Geometry check sheet. Reference: the model listing, model coordinates, mm. Face numbers are marked on the shaded views. A direction names the side the tool comes from. Coordinates: 2 decimals unless noted, no trailing zeros. Order: outer loops, then holes, each group sorted by start corner. A loop starts at its lowest first (then second) coordinate and runs counter-clockwise, first axis right, second up. Notation, with made-up numbers: (-5.5, 42) -> (52.5, 42) arc R9 ccw to (52.5, 53) -> close; hole circle Ø3 at (-39.75, 3). An arc over 180 degrees is marked (long way). Answer in a Markdown table with one row per item. Add a question column.
```python
from build123d import *

# Parameters (mm, degrees)
SCHIZZO1_W                   = 20
SCHIZZO1_H                   = 18
SCHIZZO1_R                   = 2.5
ESTRUSIONE_ESTRUSIONE1_DEPTH = 5
SCHIZZO2_W                   = 30
SCHIZZO2_H                   = 3.5
ESTRUSIONE_ESTRUSIONE2_DEPTH = 18
RACCORDO2_R                  = 1
SCHIZZO3_R                   = 2.5
TAGLIO_ESTRUSIONE1_DEPTH     = 10


with BuildPart() as part:
    # Schizzo1 → Estrusione-Estrusione1 (new body)
    with BuildSketch(Plane.XY):
        Rectangle(SCHIZZO1_W, SCHIZZO1_H)
        Circle(SCHIZZO1_R, mode=Mode.SUBTRACT)
    extrude(amount=ESTRUSIONE_ESTRUSIONE1_DEPTH)

    # Schizzo2 → Estrusione-Estrusione2 (add, through all)
    with BuildSketch(Plane.XZ.offset(9)):
        with Locations((20, 6.75)):
            Rectangle(SCHIZZO2_W, SCHIZZO2_H)
        with Locations((-20, 6.75)):
            Rectangle(SCHIZZO2_W, SCHIZZO2_H)
    extrude(amount=-ESTRUSIONE_ESTRUSIONE2_DEPTH)

    # Raccordo2
    raccordo2_edges = [part.edges().sort_by_distance(p)[0] for p in [
        (-10, 0, 5),
        (-5, 0, 5),
        (-5, 0, 8.5),
        (5, 0, 5),
        (5, 0, 8.5),
        (10, 0, 5),
        (-10, 0, 0),
        (10, 0, 0),
    ]]
    fillet(raccordo2_edges, radius=RACCORDO2_R)

    # Schizzo3 → Taglio-Estrusione1 (cut)
    with BuildSketch(Plane.XY.offset(8.5)):
        with Locations((-25, 0)):
            Circle(SCHIZZO3_R)
        with Locations((25, 0)):
            Circle(SCHIZZO3_R)
        with BuildLine():
            Line((25, 9), (35, 9))
            Line((35, 9), (35, -9))
            Line((35, -9), (25, -9))
            ThreePointArc((25, -9), (34, 0), (25, 9))
        make_face()
        with BuildLine():
            Line((-35, 9), (-35, -9))
            Line((-35, -9), (-25, -9))
            ThreePointArc((-25, -9), (-34, 0), (-25, 9))
            Line((-25, 9), (-35, 9))
        make_face()
    extrude(amount=-TAGLIO_ESTRUSIONE1_DEPTH, mode=Mode.SUBTRACT)


solid = part.part
```
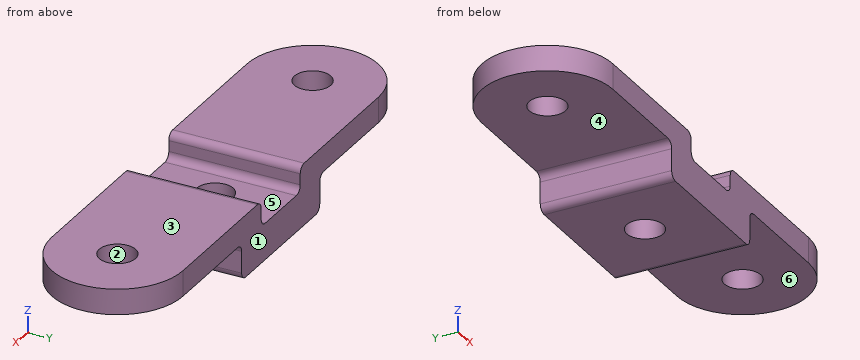
(1) Mould release check, pull along Y, two halves, no side actions. Record for the marked faces 1, 2 and 3: +Y half, -Y half, draft (parallel to the pull), parting line (faces both ways), or undercut.
(2) Cross-section at A-A (x = 0). Enter the section's corners in (y, z), plus the area to 3 significant figures.
(3) Access from +Z, -Z, +X, -X, +Y, -Y to the whole of each face (thin tool, end or side, straight path). Record for the marked faces 4, 5 and 6.
(4) Cross-section at B-B (y = 0). Give the number of separate pieces and of enclosed holes in the cut face, plus the area to 3 significant figures.
(5) Cross-section at D-D (y = -6). Enter the section's corners in (x, z).
(6) Cross-section at C-C (x = 17.5). Enter the section's corners in (y, z), plus the area to 3 significant figures.
(7) Go/stop test with flat-tipped pins: P1, Ø9, axis at x = 22, y = 2.5, coming from the -Z side; P2, Ø2.5, axis at y = -3, z = 2, coming from the +X side; P3, Ø0.8, axis at y = -3, z = 7, coming from the -X side. Record where each tip stops, or that it passes through.
(8) Scan lines: line 1 along Y through (x, z) = (0, 3.25); line 2 along X through (y, z) = (-5.75, 2.5); line 3 along Z through (x, y) = (23, -3.5). Record each from-to range of solid material in increasing order.
Checks:
| question | item | result |
|---|---|---|
| 1 | face 1 | +Y half |
| 1 | face 2 | undercut |
| 1 | face 3 | draft |
| 2 | outline | (-9, 0) -> (-2.5, 0) -> (-2.5, 5) -> (-9, 5) -> close; (2.5, 0) -> (9, 0) -> (9, 5) -> (2.5, 5) -> close |
| 2 | area | 65.0 mm² |
| 3 | face 4 | -Z, -X, +Y, -Y |
| 3 | face 5 | +Z, +Y, -Y |
| 3 | face 6 | -Z, +X, +Y, -Y |
| 4 | separate pieces | 4 |
| 4 | enclosed holes | 0 |
| 4 | area | 243 mm² |
| 5 | outline | (-31.71, 5) -> (-11, 5) arc R1 cw to (-10, 4) -> (-10, 1) arc R1 ccw to (-9, 0) -> (9, 0) arc R1 ccw to (10, 1) -> (10, 4) arc R1 cw to (11, 5) -> (31.71, 5) -> (31.71, 8.5) -> (6, 8.5) arc R1 ccw to (5, 7.5) -> (5, 6) arc R1 cw to (4, 5) -> (-4, 5) arc R1 cw to (-5, 6) -> (-5, 7.5) arc R1 ccw to (-6, 8.5) -> (-31.71, 8.5) -> close |
| 6 | outline | (-9, 5) -> (9, 5) -> (9, 8.5) -> (-9, 8.5) -> close |
| 6 | area | 63.0 mm² |
| 7 | P1 | z = 5 |
| 7 | P2 | x = 10 |
| 7 | P3 | x = -33.62 |
| 8 | line 1 | -9 to -2.5, 2.5 to 9 |
| 8 | line 2 | -10 to 10 |
| 8 | line 3 | 5 to 8.5 |
